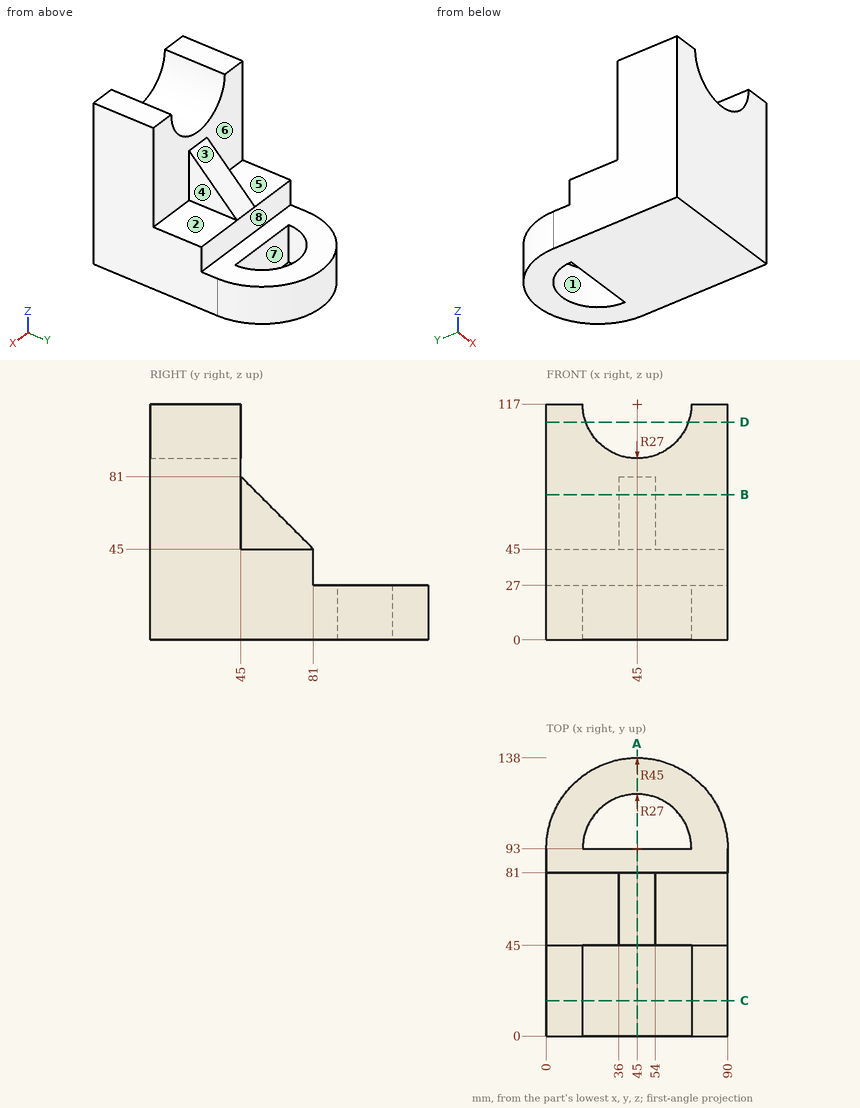
Could you check a few things on this drawing? It's one solid part, dimensions in mm from its lowest x, y, z. A direction names the side the tool comes from. Coordinates: 2 decimals unless noted, no trailing zeros. Order: outer loops, then holes, each group sorted by start corner. A loop starts at its lowest first (then second) coordinate and runs counter-clockwise, first axis right, second up. Notation, with made-up numbers: (89.25, 82.25) - (99.25, 82.25) arc R32 ccw to (99.25, 113.25) - close; hole circle Ø11 at (36.25, 75.5). An arc over 180 degrees is marked (long way). One line per question, with ' | ' between items.
(1) Suppose I cut it at D-D on z = 108. List the corners of the cut face in (x, y) for me.
Report:
outline: (0, 0) - (19.54, 0) - (19.54, 45) - (0, 45) - close; (70.46, 0) - (90, 0) - (90, 45) - (70.46, 45) - close
(2) Suppose I cut it at B-B on z = 72. List the corners of the cut face in (x, y) for me, and give its area (3 significant figures).
Report:
outline: (0, 0) - (90, 0) - (90, 45) - (54, 45) - (54, 54) - (36, 54) - (36, 45) - (0, 45) - close | area: 4,210 mm2
(3) Suppose I cut it at C-C on y = 17.5. List the corners of the cut face in (x, z) for me.
Report:
outline: (0, 0) - (90, 0) - (90, 117) - (72, 117) arc R27 cw to (18, 117) - (0, 117) - close
(4) If I drill on L1, parallel to Y at x = 66, z = 94; L2, parallel to Y at x = 34, z = 22.5, over which ranges is the centre line in solid material (lowest first)?
Report:
L1: y = 0 to 45 | L2: y = 0 to 93, 117.66 to 136.63
(5) If we mould it in two halves opening along Y, with no side actions, what happens to the marked faces 1, 2 and 3? For each: pulls with the +Y half, pulls with the -Y half, needs draft (parallel to the pull), parting line crosses it, or undercut.
Report:
face 1: undercut | face 2: needs draft | face 3: pulls with the +Y half
(6) Suppose I cut it at A-A on x = 45. List the corners of the cut face in (y, z) for me.
Report:
outline: (0, 0) - (93, 0) - (93, 27) - (81, 27) - (81, 45) - (45, 81) - (45, 90) - (0, 90) - close; (120, 0) - (138, 0) - (138, 27) - (120, 27) - close
(7) Will these pins go through, and if not, where does the flat tip stop? pin 1 (12 mm diameter, centred on x = 70, y = 85.5, fed in from +Z); pin 2 (1 mm diameter, centred on x = 78, z = 44.5, fed in from +Y); pin 3 (1 mm diameter, centred on y = 60, z = 47, fed in from +X).
Report:
pin 1: stops at z = 45 | pin 2: stops at y = 81 | pin 3: stops at x = 54
(8) For the marked faces 4, 5, 6, 7 and 8, which set-ups out of +Z, -Z, +X, -X, +Y, -Y let a thin tool reach every point of the face, with its end or its side?
Report:
face 4: +Z, +X, +Y | face 5: +Z, -X, +Y | face 6: +Z, +Y | face 7: +Z, -Z | face 8: +Z, +X, -X, +Y
